```python
from build123d import *

# Parameters (mm, degrees)
F1_DEPTH = 15.875
F2_W     = 20.955
F2_H     = 20.955
F3_DEPTH = 31.751
F5_D     = 5.5
F6_SIZE  = 2.54


with BuildPart() as f1:
    # F0 (on Top) → F1 (new body, symmetric)
    with BuildSketch(Plane.XY):
        with BuildLine():
            Line((-15.875, -28.575), (15.875, -28.575))
            Line((15.875, -28.575), (15.875, -20.32))
            Line((15.875, -20.32), (0, -20.32))
            ThreePointArc((0, -20.32), (-8.5725, -11.7475), (0, -3.175))
            Line((0, -3.175), (15.875, -3.175))
            Line((15.875, -3.175), (15.875, 28.575))
            Line((15.875, 28.575), (-15.875, 28.575))
            Line((-15.875, 28.575), (-15.875, -28.575))
        make_face()
    extrude(amount=F1_DEPTH, both=True)

    # F2 (on face) → F3 (cut, through all)
    with BuildSketch(Plane.YZ.offset(15.875)):
        with Locations((18.0975, 0)):
            Rectangle(F2_W, F2_H)
    extrude(amount=-F3_DEPTH, mode=Mode.SUBTRACT)

    # F5 (through all)
    with Locations(Plane.XY.offset(15.875)):
        with Locations((-9.525, 18.0975), (9.525, 18.0975)):
            Hole(F5_D / 2)

    # F6
    f6_edges = [f1.edges().sort_by_distance(p)[0] for p in [
        (15.875, -20.32, 0),
        (15.875, -3.175, 0),
    ]]
    chamfer(f6_edges, length=F6_SIZE)


solid = f1.part
```
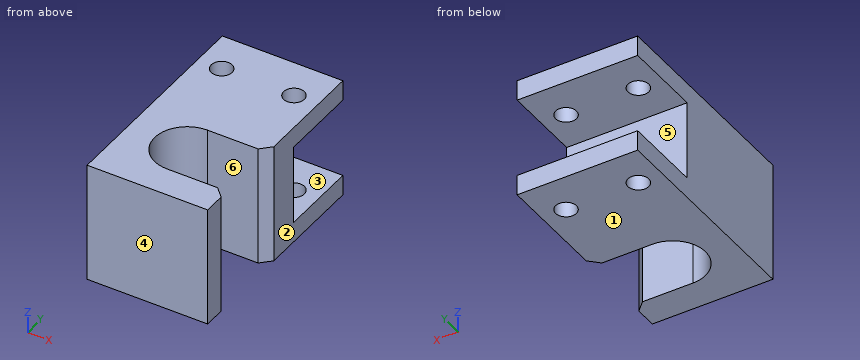
Check sheet for the modelled part. Datum: model origin and axes. Units: mm. Face numbers are marked on the shaded views. A direction names the side the tool comes from. Give positions to 0.01 mm unless a question says otherwise; leave off trailing zeros. Write each loop counter-clockwise with the first axis right and the second up, starting at its lowest first coordinate (ties: lowest second). Pieces come first, ordered by that corner, then holes.
Item 1: Scan lines: L1, parallel to Y at x = 9.5, z = 14.5 (3 decimals); L2, parallel to Z at x = -4, y = 20 (1 decimal); L3, parallel to X at y = 16, z = -13.5 (3 decimals). Record each from-to range of solid material in increasing order.
Item 2: Cross-section at D-D (z = 9). Enter the section's corners in (x, y) (1 decimal), and give its area (3 significant figures).
Item 3: Cross-section at B-B (x = 1). Enter the section's corners in (y, z) (1 decimal).
Item 4: Cross-section at C-C (x = -14). Enter the section's corners in (y, z) (1 decimal), and give its area (3 significant figures).
Item 5: Gauge pin test, flat ends, axial feed: pin 1 (1.5 mm diameter, centred on x = 1, z = 4.5, fed in from +Y); pin 2 (12 mm diameter, centred on x = -7.5, y = 18, fed in from -Z) (3 decimals); pin 3 (12 mm diameter, centred on y = -16, z = 7, fed in from +X) (3 decimals). Record the tip position at first contact, or that the pin passes through.
Item 6: Access from +Z, -Z, +X, -X, +Y, -Y to the whole of each face (thin tool, end or side, straight path). Record for the marked faces 4, 5 and 6.
Item 7: Cross-section at A-A (y = 12.5). Enter the section's corners in (x, z) (1 decimal).
Item 8: Draft check along Z on the marked faces 1, 2 and 3. Enter one of: released by +Z, released by -Z, zero draft, split by the parting line, or undercut.
Report:
1. L1: y = -28.575 to -20.32, -3.175 to 15.348, 20.847 to 28.575
1. L2: z = -15.9 to -10.5, 10.5 to 15.9
1. L3: x = -15.875 to -11.303, -7.747 to 7.747, 11.303 to 15.875
2. outline: (-15.9, -28.6) - (15.9, -28.6) - (15.9, -22.9) - (13.3, -20.3) - (0, -20.3) arc R8.6 cw to (0, -3.2) - (13.3, -3.2) - (15.9, -0.6) - (15.9, 7.6) - (-15.9, 7.6) - close
2. area: 755 mm2
3. outline: (-28.6, -15.9) - (-20.3, -15.9) - (-20.3, 15.9) - (-28.6, 15.9) - close; (-3.2, -15.9) - (28.6, -15.9) - (28.6, -10.5) - (7.6, -10.5) - (7.6, 10.5) - (28.6, 10.5) - (28.6, 15.9) - (-3.2, 15.9) - close
4. outline: (-28.6, -15.9) - (28.6, -15.9) - (28.6, -10.5) - (7.6, -10.5) - (7.6, 10.5) - (28.6, 10.5) - (28.6, 15.9) - (-28.6, 15.9) - close
4. area: 1,380 mm2
5. pin 1: stops at y = 7.62
5. pin 2: stops at z = -15.875
5. pin 3: stops at x = 15.015
6. face 4: +Z, -Z, +X, -X, -Y
6. face 5: +X, -X, +Y
6. face 6: +Z, -Z, +X
7. outline: (-15.9, -15.9) - (15.9, -15.9) - (15.9, -10.5) - (-15.9, -10.5) - close; (-15.9, 10.5) - (15.9, 10.5) - (15.9, 15.9) - (-15.9, 15.9) - close
8. face 1: released by -Z
8. face 2: zero draft
8. face 3: undercut
